from build123d import *

# Parameters (mm, degrees)
SKETCH1_W           = 34
SKETCH1_H           = 9.5
BOSS_EXTRUDE1_DEPTH = 0.45
SKETCH2_W           = 0.7
SKETCH2_H           = 9.5
BOSS_EXTRUDE2_DEPTH = 1.2
SKETCH3_R           = 2
BOSS_EXTRUDE3_DEPTH = 1
SKETCH4_W           = 3.524824873
SKETCH4_H           = 0.673444534
SKETCH4_H_2         = 0.672160641
BOSS_EXTRUDE4_DEPTH = 1.2


with BuildPart() as part:
    # Sketch1 → Boss-Extrude1 (new body)
    with BuildSketch(Plane(origin=(0, 0, 0), x_dir=(1, 0, 0), z_dir=(0, 1, 0))):
        with Locations((5.143034826, -1.016169154)):
            Rectangle(SKETCH1_W, SKETCH1_H)
    extrude(amount=BOSS_EXTRUDE1_DEPTH)

    # Sketch2 → Boss-Extrude2 (add)
    with BuildSketch(Plane(origin=(0, 0.45, 0), x_dir=(1, 0, 0), z_dir=(0, 1, 0))):
        with Locations((-11.506965174, -1.016169154)):
            Rectangle(SKETCH2_W, SKETCH2_H)
    extrude(amount=BOSS_EXTRUDE2_DEPTH)

    # Sketch3 → Boss-Extrude3 (add)
    with BuildSketch(Plane(origin=(0, 0.45, 0), x_dir=(1, 0, 0), z_dir=(0, 1, 0))):
        with Locations((-3.756965174, -1.016169154)):
            Circle(SKETCH3_R)
        with Locations((4.893034826, -1.016169154)):
            Circle(SKETCH3_R)
        with Locations((14.323034826, -1.016169154)):
            Circle(SKETCH3_R)
    extrude(amount=BOSS_EXTRUDE3_DEPTH)

    # Sketch4 → Boss-Extrude4 (add)
    with BuildSketch(Plane(origin=(0, 0.45, 0), x_dir=(1, 0, 0), z_dir=(0, 1, 0))):
        with Locations((20.38062239, 3.397108579)):
            Rectangle(SKETCH4_W, SKETCH4_H)
        with Locations((20.38062239, -5.430088834)):
            Rectangle(SKETCH4_W, SKETCH4_H_2)
    extrude(amount=BOSS_EXTRUDE4_DEPTH)


solid = part.part
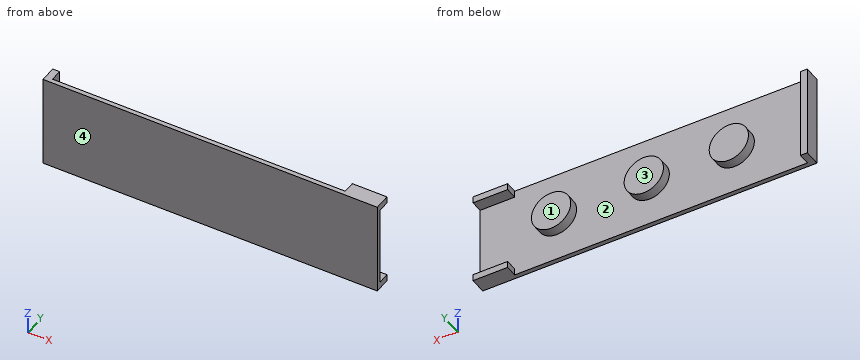
Design review of the part built by this model. Coordinates are the model's own, in mm. Face numbers are marked on the shaded views. A direction names the side the tool comes from. Coordinates: 2 decimals unless noted, no trailing zeros. Loops run counter-clockwise (first coordinate to the right, second up) from the corner with the lowest first, then second, coordinate; pieces in that order, holes last. Notation, with made-up numbers: (51.5, -37) -> (105.5, -37) arc R27 cw to (105.5, -17) -> close; hole circle Ø8 at (86, 48). An arc over 180 degrees is marked (long way). Use a Markdown table: item, result. Add a question column.
Item 1: We need section A-A, the plane y = 0.85. Write out the cut boundary in (x, z).
Item 2: We need section C-C, the plane x = 4. Write out the cut boundary in (y, z), and give its area (3 significant figures).
Item 3: Machinability: for the marked faces 3 and 4, which of the approach directions +Z, -Z, +X, -X, +Y, -Y give a long, thin tool a straight path to every point of the face, cutting with its end or side? Answer none if there is none.
Item 4: Wall thickness on L1, parallel to X at y = 1.15, z = 0; L2, parallel to X at y = 1.1, z = 0.25; L3, parallel to Z at x = 19.5, y = 1.6: over which ranges is each line inside the solid? List them lowest first. Write a range as from..to.
Item 5: We need section D-D, the plane z = -0.25. Write out the cut boundary in (x, y), and give its area (3 significant figures).
Item 6: Clearance check with flat-ended pins moving along their axes: P1, Ø1.2, axis at x = -3, z = 0, coming from the +Y side; P2, Ø3, axis at x = 9, z = -1, coming from the +Y side; P3, Ø5, axis at x = -7, z = 1.5, coming from the -Y side. State where each tip first meets the part, or that it passes through.
Item 7: We need section B-B, the plane z = 3.5. Write out the cut boundary in (x, y).
Item 8: The part is to be moulded in two halves that separate along X. For the marked faces 1 and 2, say which applies: +X half, -X half, draft (parallel to the pull), parting line (faces both ways), or undercut.
Numbers:
| question | item | result |
|---|---|---|
| 1 | outline | (-11.86, -3.73) -> (-11.16, -3.73) -> (-11.16, 5.77) -> (-11.86, 5.77) -> close; circle Ø4 at (-3.76, 1.02); circle Ø4 at (4.89, 1.02); circle Ø4 at (14.32, 1.02); (18.62, -3.73) -> (22.14, -3.73) -> (22.14, -3.06) -> (18.62, -3.06) -> close; (18.62, 5.09) -> (22.14, 5.09) -> (22.14, 5.77) -> (18.62, 5.77) -> close |
| 2 | outline | (0, -3.73) -> (0.45, -3.73) -> (0.45, -0.77) -> (1.45, -0.77) -> (1.45, 2.81) -> (0.45, 2.81) -> (0.45, 5.77) -> (0, 5.77) -> close |
| 2 | area | 7.85 mm^2 |
| 3 | face 3 | +Z, -Z, +X, +Y |
| 3 | face 4 | +Z, -Z, +X, -X, -Y |
| 4 | L1 | x = -11.86..-11.16, -5.48..-2.03, 3.17..6.62, 12.6..16.05 |
| 4 | L2 | x = -11.86..-11.16, -5.6..-1.91, 3.05..6.74, 12.48..16.17 |
| 4 | L3 | z = -3.73..-3.06, 5.09..5.77 |
| 5 | outline | (-11.86, 0) -> (22.14, 0) -> (22.14, 0.45) -> (15.87, 0.45) -> (15.87, 1.45) -> (12.77, 1.45) -> (12.77, 0.45) -> (6.44, 0.45) -> (6.44, 1.45) -> (3.34, 1.45) -> (3.34, 0.45) -> (-2.21, 0.45) -> (-2.21, 1.45) -> (-5.31, 1.45) -> (-5.31, 0.45) -> (-11.16, 0.45) -> (-11.16, 1.65) -> (-11.86, 1.65) -> close |
| 5 | area | 25.4 mm^2 |
| 6 | P1 | stops at y = 1.45 |
| 6 | P2 | stops at y = 0.45 |
| 6 | P3 | stops at y = 0 |
| 7 | outline | (-11.86, 0) -> (22.14, 0) -> (22.14, 0.45) -> (-11.16, 0.45) -> (-11.16, 1.65) -> (-11.86, 1.65) -> close |
| 8 | face 1 | draft |
| 8 | face 2 | undercut |
